Answer from the drawing. Dimensions are ordinates in mm from the lowest x, y and z of the part. A direction names the side the tool comes from. Coordinates: 2 decimals unless noted, no trailing zeros. Order: outer loops, then holes, each group sorted by start corner. A loop starts at its lowest first (then second) coordinate and runs counter-clockwise, first axis right, second up. Notation, with made-up numbers: (42.25, 42.25) - (79.25, 42.25) arc R35 ccw to (79.25, 79.25) - close; hole circle Ø8 at (72.25, -27.75). An arc over 180 degrees is marked (long way). Answer as a JSON object with one key per item and string values. Group by question number.
1) Section A-A (x = 25) is taken. Give the vertices of the cut face in (y, z), plus the area to 3 significant figures.
2) A tool of negligible diameter and unlimited length cuts with its end or side. For the marked faces 1 and 2, from which of +Z, -Z, +X, -X, +Y, -Y can it reach the whole face along a straight path? Write none if from no direction.
3) The mould has two halves that part along Y. Classify the marked faces 3, 4 and 5: released by +Y, released by -Y, zero draft, split by the parting line, or undercut.
4) Section C-C (y = 4) is taken. Give the vertices of the cut face in (x, z), plus the area to 3 significant figures.
5) Section B-B (z = 7.25) is taken. Give the vertices of the cut face in (x, y).
6) Find the intervals of material crossed by line 1 along Y through (x, z) = (25, 3); line 2 along Y through (x, z) = (25, 6); line 3 along X through (y, z) = (3.25, 5.75), in increasing order.
7) Section D-D (z = 3.5) is taken. Give the vertices of the cut face in (x, y), plus the area to 3 significant figures.
8) This flat-tipped pin is pushed along its axis until it touches: P1, Ø4, axis at x = 25, y = 18, coming from the +Z side. Where does it stop, or does it pass through?
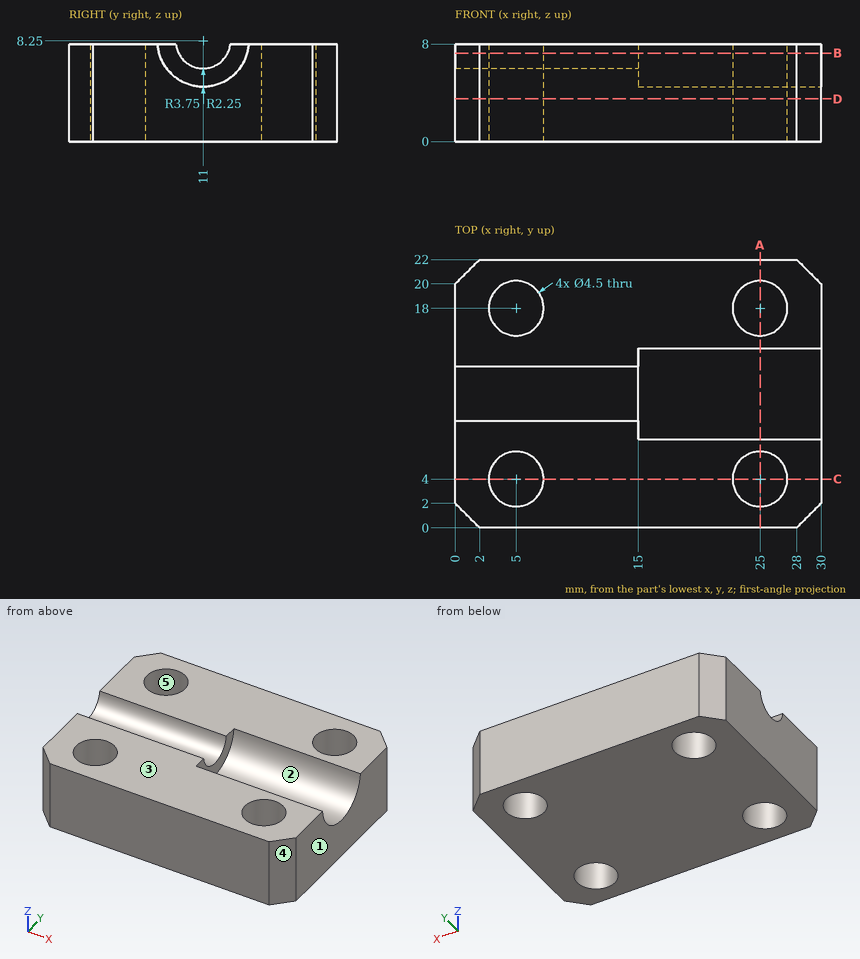
Report:
{
 "1": {"outline": "(0, 0) - (1.75, 0) - (1.75, 8) - (0, 8) - close; (6.25, 0) - (15.75, 0) - (15.75, 8) - (14.74, 8) arc R3.75 cw to (7.26, 8) - (6.25, 8) - close; (20.25, 0) - (22, 0) - (22, 8) - (20.25, 8) - close", "area": "83.8 mm²"},
 "2": {"face 1": "+Z, -Z, +X, +Y, -Y", "face 2": "+Z, +X"},
 "3": {"face 3": "zero draft", "face 4": "released by -Y", "face 5": "undercut"},
 "4": {"outline": "(0, 0) - (2.75, 0) - (2.75, 8) - (0, 8) - close; (7.25, 0) - (22.75, 0) - (22.75, 8) - (7.25, 8) - close; (27.25, 0) - (30, 0) - (30, 8) - (27.25, 8) - close", "area": "168 mm²"},
 "5": {"outline": "(0, 2) - (2, 0) - (28, 0) - (30, 2) - (30, 7.39) - (15, 7.39) - (15, 8.98) - (0, 8.98) - close; (0, 13.02) - (15, 13.02) - (15, 14.61) - (30, 14.61) - (30, 20) - (28, 22) - (2, 22) - (0, 20) - close; hole circle Ø4.5 at (5, 4); hole circle Ø4.5 at (5, 18); hole circle Ø4.5 at (25, 4); hole circle Ø4.5 at (25, 18)"},
 "6": {"line 1": "y = 0 to 1.75, 6.25 to 15.75, 20.25 to 22", "line 2": "y = 0 to 1.75, 6.25 to 8, 14 to 15.75, 20.25 to 22", "line 3": "x = 0 to 2.88, 7.12 to 22.88, 27.12 to 30"},
 "7": {"outline": "(0, 2) - (2, 0) - (28, 0) - (30, 2) - (30, 20) - (28, 22) - (2, 22) - (0, 20) - close; hole circle Ø4.5 at (5, 4); hole circle Ø4.5 at (5, 18); hole circle Ø4.5 at (25, 4); hole circle Ø4.5 at (25, 18)", "area": "588 mm²"},
 "8": {"P1": "passes through"}
}
